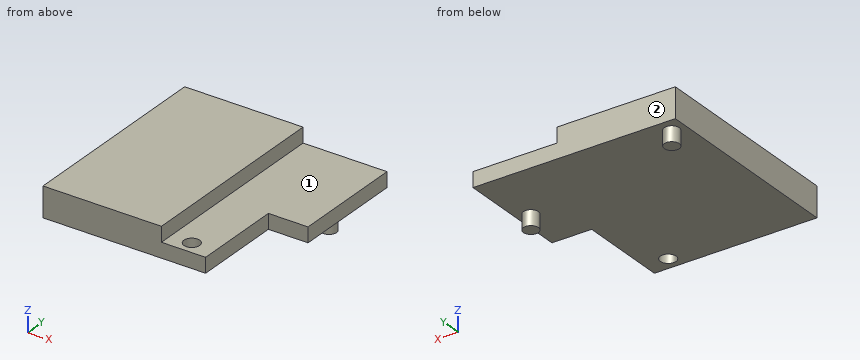
from build123d import *

# Parameters (mm, degrees)
SKETCH1_W           = 27
SKETCH1_H           = 27.3
SKETCH1_R           = 1.05
BOSS_EXTRUDE1_DEPTH = 2
SKETCH2_W           = 5.3
SKETCH2_H           = 12
CUT_EXTRUDE1_DEPTH  = 79.521414277
SKETCH3_R           = 1
BOSS_EXTRUDE2_DEPTH = 4
SKETCH4_W           = 15.8
SKETCH4_H           = 27.3
BOSS_EXTRUDE3_DEPTH = 2
SKETCH5_W           = 27
SKETCH5_H           = 0.2
CUT_EXTRUDE2_DEPTH  = 79.597789409


with BuildPart() as part:
    # Sketch1 → Boss-Extrude1 (new body)
    with BuildSketch(Plane.XY):
        with Locations((40.15, -43.65)):
            Rectangle(SKETCH1_W, SKETCH1_H)
        with Locations((45.25, -55.5)):
            Circle(SKETCH1_R, mode=Mode.SUBTRACT)
    extrude(amount=BOSS_EXTRUDE1_DEPTH)

    # Sketch2 → Cut-Extrude1 (cut, through all)
    with BuildSketch(Plane.XY.offset(2)):
        with Locations((51, -51.3)):
            Rectangle(SKETCH2_W, SKETCH2_H)
    extrude(amount=-CUT_EXTRUDE1_DEPTH, mode=Mode.SUBTRACT)

    # Sketch3 → Boss-Extrude2 (add)
    with BuildSketch(Plane.XY.offset(2)):
        with Locations((28.45, -32.1)):
            Circle(SKETCH3_R)
        with Locations((51.85, -38.7)):
            Circle(SKETCH3_R)
    extrude(amount=-BOSS_EXTRUDE2_DEPTH)

    # Sketch4 → Boss-Extrude3 (add)
    with BuildSketch(Plane.XY.offset(2)):
        with Locations((34.55, -43.65)):
            Rectangle(SKETCH4_W, SKETCH4_H)
    extrude(amount=BOSS_EXTRUDE3_DEPTH)

    # Sketch5 → Cut-Extrude2 (cut, through all)
    with BuildSketch(Plane(origin=(0, 0, 0), x_dir=(-1, 0, 0), z_dir=(0, 0, -1))):
        with Locations((-40.15, -30.1)):
            Rectangle(SKETCH5_W, SKETCH5_H)
    extrude(amount=-CUT_EXTRUDE2_DEPTH, mode=Mode.SUBTRACT)


solid = part.part
Input: part model. Units: mm. Frame: model coordinates. Face numbers are marked on the shaded views. A direction names the side the tool comes from. Coordinates: 2 decimals unless noted, no trailing zeros. Order: outer loops, then holes, each group sorted by start corner. A loop starts at its lowest first (then second) coordinate and runs counter-clockwise, first axis right, second up.
1. Cut plane C-C, the plane y = -55.5. Return loops of the section in (x, z), plus the area to 3 significant figures.
Checked values:
outline: (26.65, 0) - (44.2, 0) - (44.2, 2) - (42.45, 2) - (42.45, 4) - (26.65, 4) - close; (46.3, 0) - (48.35, 0) - (48.35, 2) - (46.3, 2) - close
area: 70.8 mm2
2. Cut plane A-A, the plane z = 1.45. Return loops of the section in (x, y).
Checked values:
outline: (26.65, -57.3) - (48.35, -57.3) - (48.35, -45.3) - (53.65, -45.3) - (53.65, -30.2) - (26.65, -30.2) - close; hole circle Ø2.1 at (45.25, -55.5)
3. Ray query, line 1 along Y through (x, z) = (45.25, 0.75); line 2 along Z through (x, y) = (32.5, -50.75); line 3 along Y through (x, z) = (49.5, 0.4). Return the intervals inside material, ascending.
Checked values:
line 1: y = -57.3 to -56.55, -54.45 to -30.2
line 2: z = 0 to 4
line 3: y = -45.3 to -30.2
4. Access query for the marked faces 1 and 2. Directions: +Z, -Z, +X, -X, +Y, -Y. A direction counts if a zero-diameter tool reaches every point of the face in a straight line with its end or side. Return the directions, or none.
Checked values:
face 1: +Z, +X, +Y, -Y
face 2: +Z, -Z, +X, -X, +Y
5. Cut plane B-B, the plane x = 45.25. Return loops of the section in (y, z), plus the area to 3 significant figures.
Checked values:
outline: (-57.3, 0) - (-56.55, 0) - (-56.55, 2) - (-57.3, 2) - close; (-54.45, 0) - (-30.2, 0) - (-30.2, 2) - (-54.45, 2) - close
area: 50.0 mm2
6. Cut plane D-D, the plane x = 51.85. Return loops of the section in (y, z), plus the area to 3 significant figures.
Checked values:
outline: (-45.3, 0) - (-39.7, 0) - (-39.7, -2) - (-37.7, -2) - (-37.7, 0) - (-30.2, 0) - (-30.2, 2) - (-45.3, 2) - close
area: 34.2 mm2
7. Contact query for flat-ended pins moving along their axis: P1, Ø10, axis at x = 51, y = -37, coming from the +Z side; P2, Ø0.6, axis at y = -52, z = 0.5, coming from the +X side; P3, Ø0.6, axis at x = 52, z = 0.5, coming from the -Y side. Output: stop coordinate, or through.
Checked values:
P1: stops at z = 2
P2: stops at x = 48.35
P3: stops at y = -45.3
